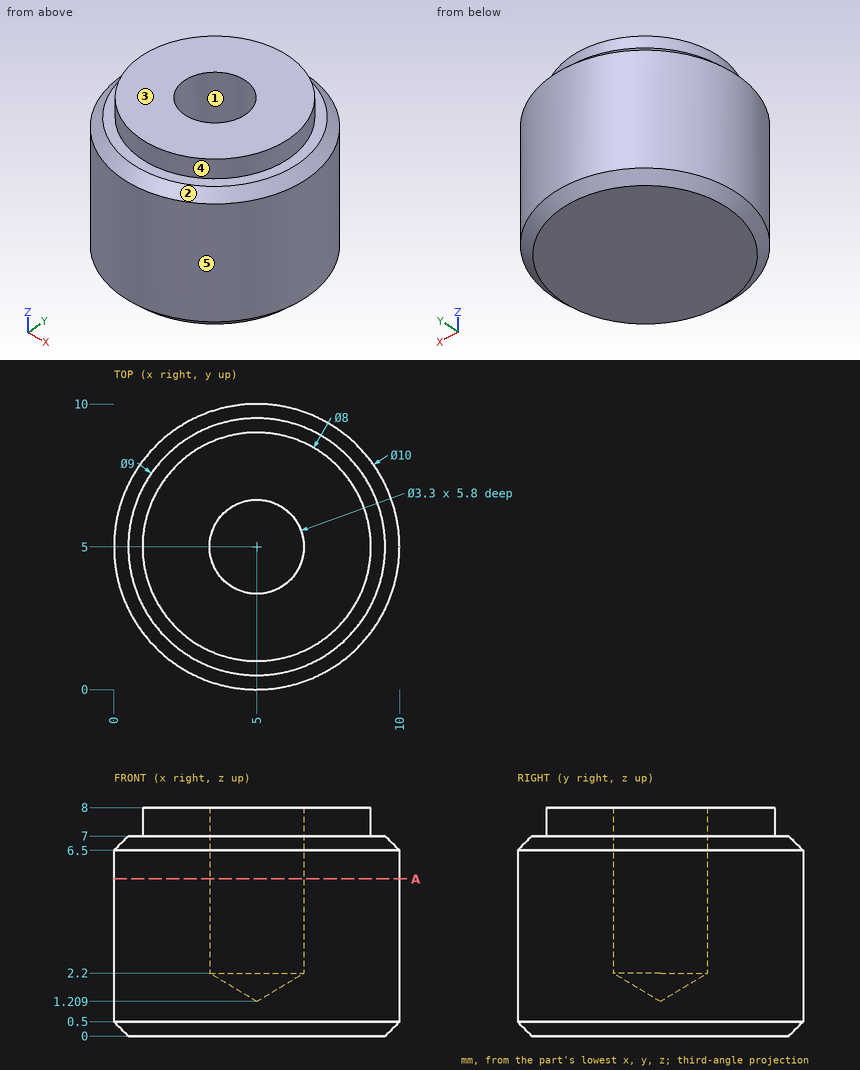
Print and shaded views of the part. All mm, measured from the part's lowest x, y and z. A direction names the side the tool comes from. Round coordinates to 2 decimals unless told otherwise and drop trailing zeros. Order: outer loops, then holes, each group sorted by start corner. A loop starts at its lowest first (then second) coordinate and runs counter-clockwise, first axis right, second up.
Q1. Two-plate mould, pull along Y, no slides. Class the marked faces 1, 2 and 3: pulls with the +Y half, pulls with the -Y half, needs draft (parallel to the pull), parting line crosses it, or undercut.
Q2. Wall check: L1, parallel to Y at x = 5, z = 6.2; L2, parallel to Y at x = 4.25, z = 4 (1 decimal); L3, parallel to X at y = 5.5, z = 7.5. Give the ranges that are in metal, low to high.
Q3. Drop a flat-ended pin along its axis: pin 1 (1.5 mm diameter, centred on y = 3, z = 3.5, fed in from -X). Give the stop position or say it passes through.
Q4. Which spindle directions (+Z, -Z, +X, -X, +Y, -Y) get a long thin tool onto all of the face, cutting with end or side? Do the marked faces 4 and 5. Say none if no direction does.
Q5. Slice it at A-A (z = 5.5). Write the cut outline in (x, y).
Results below:
1. face 1: undercut
1. face 2: parting line crosses it
1. face 3: needs draft
2. L1: y = 0 to 3.35, 6.65 to 10
2. L2: y = 0.1 to 3.5, 6.5 to 9.9
2. L3: x = 1.03 to 3.43, 6.57 to 8.97
3. pin 1: stops at x = 0.16
4. face 4: +Z
4. face 5: +Z, -Z
5. outline: circle Ø10 at (5, 5); hole circle Ø3.3 at (5, 5)
